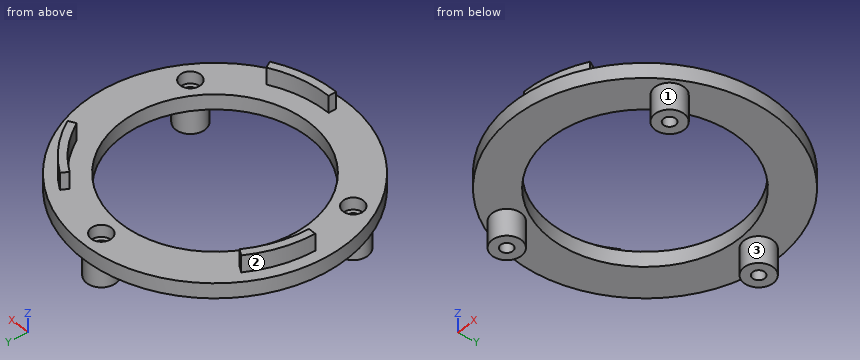
from build123d import *

# Parameters (mm, degrees)
SKETCH1_R           = 35
SKETCH1_R_2         = 30
SKETCH1_R_3         = 25
BOSS_EXTRUDE1_DEPTH = 4
SKETCH2_R           = 3.9
BOSS_EXTRUDE2_DEPTH = 7.1
SKETCH3_R           = 1.6
CUT_EXTRUDE1_DEPTH  = 15
SKETCH4_R           = 2.7
CUT_EXTRUDE2_DEPTH  = 3.2
BOSS_EXTRUDE3_DEPTH = 4.5
BOSS_EXTRUDE4_DEPTH = 4.5


with BuildPart() as part:
    # Sketch1 → Boss-Extrude1 (new body)
    with BuildSketch(Plane.XY):
        Circle(SKETCH1_R)
        Circle(SKETCH1_R_2, mode=Mode.SUBTRACT)
        Circle(SKETCH1_R_2)
        Circle(SKETCH1_R_3, mode=Mode.SUBTRACT)
    extrude(amount=BOSS_EXTRUDE1_DEPTH)

    # Sketch2 → Boss-Extrude2 (add)
    with BuildSketch(Plane(origin=(0, 0, 0), x_dir=(-1, 0, 0), z_dir=(0, 0, -1))):
        with Locations((0, 30)):
            Circle(SKETCH2_R)
        with Locations((25.980762114, -15)):
            Circle(SKETCH2_R)
        with Locations((-25.980762114, -15)):
            Circle(SKETCH2_R)
    extrude(amount=BOSS_EXTRUDE2_DEPTH)

    # Sketch3 → Cut-Extrude1 (cut)
    with BuildSketch(Plane(origin=(0, 0, -7.1), x_dir=(-1, 0, 0), z_dir=(0, 0, -1))):
        with Locations((0, 30)):
            Circle(SKETCH3_R)
        with Locations((25.980762114, -15)):
            Circle(SKETCH3_R)
        with Locations((-25.980762114, -15)):
            Circle(SKETCH3_R)
    extrude(amount=-CUT_EXTRUDE1_DEPTH, mode=Mode.SUBTRACT)

    # Sketch4 → Cut-Extrude2 (cut)
    with BuildSketch(Plane.XY.offset(4)):
        with Locations((0, 30)):
            Circle(SKETCH4_R)
        with Locations((25.980762114, -15)):
            Circle(SKETCH4_R)
        with Locations((-25.980762114, -15)):
            Circle(SKETCH4_R)
    extrude(amount=-CUT_EXTRUDE2_DEPTH, mode=Mode.SUBTRACT)

    # Sketch6 → Boss-Extrude3 (add)
    with BuildSketch(Plane.XY.offset(4)):
        with BuildLine():
            Line((25.980762114, 15), (27.712812921, 16))
            ThreePointArc((27.712812921, 16), (22.627416998, 22.627416998), (16, 27.712812921))
            Line((16, 27.712812921), (15, 25.980762114))
            ThreePointArc((15, 25.980762114), (21.213203436, 21.213203436), (25.980762114, 15))
        make_face()
    extrude(amount=BOSS_EXTRUDE3_DEPTH)

    # Sketch7 → Boss-Extrude4 (add)
    with BuildSketch(Plane.XY.offset(4)):
        with BuildLine():
            Line((16, -27.712812921), (15, -25.980762114))
            ThreePointArc((15, -25.980762114), (7.764571353, -28.977774789), (0, -30))
            Line((0, -30), (0, -32))
            ThreePointArc((0, -32), (8.282209443, -30.909626441), (16, -27.712812921))
        make_face()
        with BuildLine():
            Line((25.980762114, 15), (27.712812921, 16))
            ThreePointArc((27.712812921, 16), (22.627416998, 22.627416998), (16, 27.712812921))
            Line((16, 27.712812921), (15, 25.980762114))
            ThreePointArc((15, 25.980762114), (21.213203436, 21.213203436), (25.980762114, 15))
        make_face()
        with BuildLine():
            Line((-32, 0), (-30, 0))
            ThreePointArc((-30, 0), (-28.977774789, 7.764571353), (-25.980762114, 15))
            Line((-25.980762114, 15), (-27.712812921, 16))
            ThreePointArc((-27.712812921, 16), (-30.909626441, 8.282209443), (-32, 0))
        make_face()
    extrude(amount=BOSS_EXTRUDE4_DEPTH)


solid = part.part
Can you work these out from the model? Positions are in its coordinate system, mm. Face numbers are marked on the shaded views. Round coordinates to 2 decimals unless told otherwise and drop trailing zeros. Write each loop counter-clockwise with the first axis right and the second up, starting at its lowest first coordinate (ties: lowest second). Pieces come first, ordered by that corner, then holes. Notation, with made-up numbers: (39.5, -11.5) -> (48.5, -11.5) arc R9 ccw to (48.5, -6.5) -> close; hole circle Ø4 at (-10, 0.25). An arc over 180 degrees is marked (long way). Use one line per item in the form item = value. Start each with the question number.
Q1. Imagine slicing it at D-D (x = 21). Please give me the cut outline in (y, z).
Q2. Imagine slicing it at B-B (y = -15). Count the separate pieces of the cut face and the enclosed holes in it, then the cut area to 3 significant figures.
Q3. We'd pull the mould along X, two halves only. Please class the marked faces 1, 2 and 3: +X half, -X half, draft (parallel to the pull), parting line (faces both ways), or undercut.
Q4. Imagine slicing it at C-C (z = -6). Please give me the cut outline in (x, y), then the cut area to 3 significant figures.
Q5. Imagine slicing it at A-A (z = 5.5). Please give me the cut outline in (x, y).
Q6. I'm going to push flat-ended pins straight in: P1, Ø5, axis at x = 0, y = 30, coming from the +Z side; P2, Ø1.5, axis at x = 25, z = -1, coming from the +Y side; P3, Ø2.5, axis at x = 1.5, y = 30, coming from the +Z side. Where does each tip first touch, or does it pass through?
Q7. If I drill on probe 1 along Y at (x, z) = (0, 1.75); probe 2 along Y at (x, z) = (0, -3.75); probe 3 along Z at (x, y) = (-21, -17), over which ranges is the centre line in solid material (lowest first)? Write a range as [from, to].
Worked out:
q1.outline = (-28, 0) -> (-13.56, 0) -> (-13.56, 4) -> (-28, 4) -> close; (13.56, 0) -> (28, 0) -> (28, 4) -> (24.15, 4) -> (24.15, 8.5) -> (21.42, 8.5) -> (21.42, 4) -> (13.56, 4) -> close
q2.separate_pieces = 4
q2.enclosed_holes = 0
q2.area = 119 mm^2
q3.face_1 = undercut
q3.face_2 = -X half
q3.face_3 = parting line
q4.outline = circle Ø7.8 at (-25.98, -15); circle Ø7.8 at (0, 30); circle Ø7.8 at (25.98, -15); hole circle Ø3.2 at (-25.98, -15); hole circle Ø3.2 at (0, 30); hole circle Ø3.2 at (25.98, -15)
q4.area = 119 mm^2
q5.outline = (-32, 0) -> (-30, 0) arc R30 cw to (-25.98, 15) -> (-27.71, 16) arc R32 ccw to start; (0, -32) arc R32 ccw to (16, -27.71) -> (15, -25.98) arc R30 cw to (0, -30) -> close; (15, 25.98) arc R30 cw to (25.98, 15) -> (27.71, 16) arc R32 ccw to (16, 27.71) -> close
q6.P1 = 0.8
q6.P2 = -11.11
q6.P3 = 4
q7.probe_1 = [-35, -25], [25, 27.3], [32.7, 35]
q7.probe_2 = [26.1, 28.4], [31.6, 33.9]
q7.probe_3 = [0, 4]
